from build123d import *

# Parameters (mm, degrees)
SKETCH1_W           = 313
SKETCH1_H           = 342
BOSS_EXTRUDE1_DEPTH = 6.35
SKETCH3_W           = 22
SKETCH3_H           = 155.14040353
SKETCH3_R           = 2.5
BOSS_EXTRUDE2_DEPTH = 6.35
SKETCH2_R           = 2.5
CUT_EXTRUDE1_DEPTH  = 7.35
SKETCH4_R           = 4.25
SKETCH4_R_2         = 2.5
SKETCH4_R_3         = 1.05
CUT_EXTRUDE2_DEPTH  = 7.35


with BuildPart() as part:
    # Sketch1 → Boss-Extrude1 (new body)
    with BuildSketch(Plane(origin=(0, 0, 0), x_dir=(1, 0, 0), z_dir=(0, 1, 0))):
        Rectangle(SKETCH1_W, SKETCH1_H)
    extrude(amount=-BOSS_EXTRUDE1_DEPTH)

    # Sketch3 → Boss-Extrude2 (add)
    with BuildSketch(Plane(origin=(0, 0, 0), x_dir=(1, 0, 0), z_dir=(0, 1, 0))):
        with Locations((167.5, 9)):
            Rectangle(SKETCH3_W, SKETCH3_H)
        with Locations((166.5, 9)):
            Circle(SKETCH3_R, mode=Mode.SUBTRACT)
        with Locations((166.5, -41.8)):
            Circle(SKETCH3_R, mode=Mode.SUBTRACT)
        with Locations((166.5, 59.8)):
            Circle(SKETCH3_R, mode=Mode.SUBTRACT)
    extrude(amount=-BOSS_EXTRUDE2_DEPTH)

    # Sketch2 → Cut-Extrude1 (cut, through all)
    with BuildSketch(Plane(origin=(0, 0, 0), x_dir=(1, 0, 0), z_dir=(0, 1, 0))):
        with Locations((0, -143)):
            Circle(SKETCH2_R)
        with Locations((-70, -143)):
            Circle(SKETCH2_R)
        with Locations((70, -143)):
            Circle(SKETCH2_R)
        with Locations((-70, 161)):
            Circle(SKETCH2_R)
        with Locations((0, 161)):
            Circle(SKETCH2_R)
        with Locations((70, 161)):
            Circle(SKETCH2_R)
    extrude(amount=-CUT_EXTRUDE1_DEPTH, mode=Mode.SUBTRACT)

    # Sketch4 → Cut-Extrude2 (cut, through all)
    with BuildSketch(Plane(origin=(0, 0, 0), x_dir=(1, 0, 0), z_dir=(0, 1, 0))):
        with Locations((107.204882136, 138.829587854)):
            Circle(SKETCH4_R)
        with Locations((107.204882136, 54.425387854)):
            Circle(SKETCH4_R)
        with Locations((-107.911484214, -115.605535397)):
            Circle(SKETCH4_R_2)
        with Locations((-107.911484214, 24.394464603)):
            Circle(SKETCH4_R_2)
        with Locations((112.088515786, 24.394464603)):
            Circle(SKETCH4_R_2)
        with Locations((112.088515786, -115.605535397)):
            Circle(SKETCH4_R_2)
        with Locations((-107.911484214, 138.829587854)):
            Circle(SKETCH4_R_3)
        with Locations((37.088515786, 138.829587854)):
            Circle(SKETCH4_R_3)
        with Locations((37.088515786, 43.829587854)):
            Circle(SKETCH4_R_3)
        with Locations((-107.911484214, 43.829587854)):
            Circle(SKETCH4_R_3)
    extrude(amount=-CUT_EXTRUDE2_DEPTH, mode=Mode.SUBTRACT)


solid = part.part
Verification items for the finished model (mm, model axes). Coordinates: 2 decimals unless noted, no trailing zeros. Loops run counter-clockwise (first coordinate to the right, second up) from the corner with the lowest first, then second, coordinate; pieces in that order, holes last. Notation, with made-up numbers: (-39, 83.25) -> (-4, 83.25) arc R12 ccw to (-4, 93.25) -> close; hole circle Ø5 at (81.25, 7.25). An arc over 180 degrees is marked (long way). Answer as a JSON object with one key per item and string values. Group by question number.
Item 1: Sectioned sample at A-A on y = -3. State how many separate pieces and enclosed holes the cut face has, plus the area to 3 significant figures.
Item 2: Mould release check, pull along Z, two halves, no side actions. Record for faces 1 (the flat face through (9, 0, -2)), 2 (the cylindrical face through (111.13, -3.13, -137.2)): +Z half, -Z half, draft (parallel to the pull), parting line (faces both ways), or undercut.
Item 3: Sectioned sample at B-B on z = 89.5. Record the boundary of the cut face in (x, y), plus the area to 3 significant figures.
Item 4: Scan lines: probe 1 along Z at (x, y) = (70, -3.5); probe 2 along X at (y, z) = (-4.5, -161); probe 3 along X at (y, z) = (-4.5, -55). Record each from-to range of solid material in increasing order.
Item 5: Depth check by flat-ended pin: pin 1 (3 mm diameter, centred on x = 171.5, y = -3, fed in from -Z); pin 2 (3 mm diameter, centred on x = 166.5, z = -9, fed in from +Y). Enter the tip coordinate at first touch or a pass-through.
Evaluation:
{
 "1": {"separate pieces": "1", "enclosed holes": "19", "area": "110,000 mm²"},
 "2": {"face 1": "draft", "face 2": "undercut"},
 "3": {"outline": "(-156.5, -6.35) -> (156.5, -6.35) -> (156.5, 0) -> (-156.5, 0) -> close", "area": "1,990 mm²"},
 "4": {"probe 1": "z = -171 to -163.5, -158.5 to 140.5, 145.5 to 171", "probe 2": "x = -156.5 to -72.5, -67.5 to -2.5, 2.5 to 67.5, 72.5 to 156.5", "probe 3": "x = -156.5 to 102.99, 111.42 to 178.5"},
 "5": {"pin 1": "stops at z = -86.57", "pin 2": "passes through"}
}
